Read the model definition and answer for the solid it produces. Units are mm, in the model's axes. Face numbers are marked on the shaded views. A direction names the side the tool comes from. Give positions to 0.01 mm unless a question says otherwise; leave off trailing zeros. Return JSON: item names as keys, results as strings.
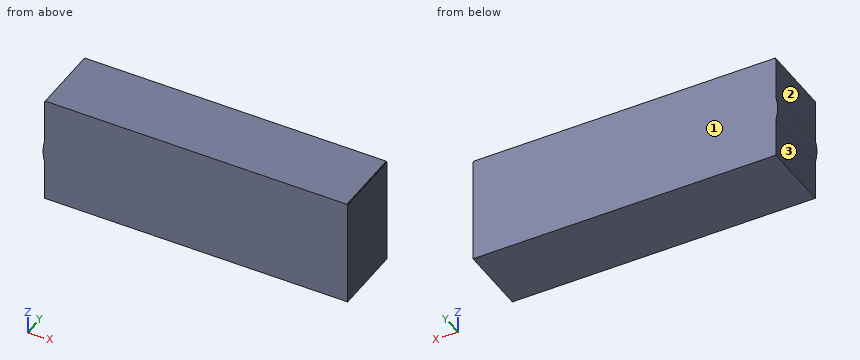
```python
from build123d import *

# Parameters (mm, degrees)
F0_W     = 109.224658
F0_H     = 38.463522
F1_DEPTH = 25.4
F2_W     = 108.63743
F2_H     = 38.757138
F3_DEPTH = 25.4
F5_DEPTH = 25.4


with BuildPart() as f1:
    # F0 (on Front) → F1 (new body)
    with BuildSketch(Plane.XZ):
        with Locations((-0.734037, 22.755137)):
            Rectangle(F0_W, F0_H)
    extrude(amount=F1_DEPTH)

    # F2 (on Front) → F3 (join)
    with BuildSketch(Plane.XZ):
        with Locations((-0.734039, 22.901945)):
            Rectangle(F2_W, F2_H)
    extrude(amount=F3_DEPTH)

    # F4 (on Front) → F5 (join)
    with BuildSketch(Plane.XZ):
        with BuildLine():
            ThreePointArc((-51.677901, 32.926388), (-55.960342, 22.03506), (-51.677901, 11.143731))
            Line((-51.677901, 11.143731), (-51.677901, 32.926388))
        make_face()
        with BuildLine():
            Line((-29.331109, 33.973895), (-29.331109, 10.096224))
            ThreePointArc((-29.331109, 10.096224), (-23.978503, 22.03506), (-29.331109, 33.973895))
        make_face()
    extrude(amount=F5_DEPTH)


solid = f1.part
```
Q1. Consider L1, parallel to X at y = -2.5, z = 21.5; L2, parallel to X at y = -9, z = 40. Determine where each line is inside the solid, lowest interval first.
Values:
{"L1": "x = -55.95 to 53.88", "L2": "x = -55.35 to 53.88"}
Q2. For the marked faces 1, 2 and 3, determine the directions among +Z, -Z, +X, -X, +Y, -Y from which every point of the face is accessible in a straight line to the end or side of a thin tool.
Values:
{"face 1": "+Z, -Z, +X, -X, +Y", "face 2": "+Z, -X, +Y, -Y", "face 3": "-Z, -X, +Y, -Y"}
Q3. Given pin 1 (8 mm diameter, centred on y = -17, z = 34, fed in from -X); pin 2 (1 mm diameter, centred on x = 1.5, z = 20, fed in from +Y), each flat-ended and moving along its own axis, determine where each tip first touches the part or whether it passes through.
Values:
{"pin 1": "stops at x = -55.35", "pin 2": "stops at y = 0"}
